```python
from build123d import *

# Parameters (mm, degrees)
SKETCH1_R           = 2.992461664
BOSS_EXTRUDE1_DEPTH = 8
CHAMFER2_SIZE       = 0.3


with BuildPart() as part:
    # Sketch1 → Boss-Extrude1 (new body)
    with BuildSketch(Plane(origin=(0, 0, 0), x_dir=(1, 0, 0), z_dir=(0, 1, 0))):
        Circle(SKETCH1_R)
        with BuildLine():
            Line((-1.125, 1.307669683), (-1.125, -1.307669683))
            ThreePointArc((-1.125, -1.307669683), (1.725, 0), (-1.125, 1.307669683))
        make_face(mode=Mode.SUBTRACT)
    extrude(amount=BOSS_EXTRUDE1_DEPTH)

    # Chamfer2
    chamfer2_edges = [part.edges().sort_by_distance(p)[0] for p in [
        (1.725, 8, 0),
        (-1.125, 8, 0),
    ]]
    chamfer(chamfer2_edges, length=CHAMFER2_SIZE)


solid = part.part
```
The model under review builds one solid part; all positions refer to its coordinate system, in mm. Coordinates: 2 decimals unless noted, no trailing zeros. Write each loop counter-clockwise with the first axis right and the second up, starting at its lowest first coordinate (ties: lowest second). Pieces come first, ordered by that corner, then holes.
1) We need section B-B on x = 0. State the section outline as (y, z) points (3 decimals).
2) We need section A-A on z = 0. State the section outline as (x, y) points (3 decimals).
3) We need section C-C on y = 3. State the section outline as (x, z) points (3 decimals), then the cut area to 3 significant figures.
4) To check wall thickness, follow probe 1 along Z at (x, y) = (0, 4.75) (3 decimals); probe 2 along X at (y, z) = (5.25, 0) (3 decimals); probe 3 along X at (y, z) = (7.5, -1.4). State the ranges of each line that lie inside material, in increasing order.
5) The part is to be moulded in two halves that separate along X. For faces 1 (the face through (2, 8, 1)), 2 (the face through (-1.125, 4, 0)), 3 (the face through (2.854, 3.944, -0.899)), say which applies: pulls with the +X half, pulls with the -X half, needs draft (parallel to the pull), parting line crosses it, or undercut.
6) Clearance check with a flat-ended pin moving along its axis: pin 1 Ø1 at (y, z) = (6, 2) entering from +X. State where the tip first meets the part, or that it passes through.
7) We need section D-D on z = 2.65. State the section outline as (x, y) points, then the cut area to 3 significant figures.
Answer list:
1. outline: (0, -2.992) - (8, -2.992) - (8, -2.025) - (7.7, -1.725) - (0, -1.725) - close; (0, 1.725) - (7.7, 1.725) - (8, 2.025) - (8, 2.992) - (0, 2.992) - close
2. outline: (-2.992, 0) - (-1.125, 0) - (-1.125, 7.7) - (-1.425, 8) - (-2.992, 8) - close; (1.725, 0) - (2.992, 0) - (2.992, 8) - (2.025, 8) - (1.725, 7.7) - close
3. outline: circle Ø5.985 at (0, 0); hole (-1.125, -1.308) arc R1.725 ccw (long way) to (-1.125, 1.308) - close
3. area: 19.9 mm2
4. probe 1: z = -2.992 to -1.725, 1.725 to 2.992
4. probe 2: x = -2.992 to -1.125, 1.725 to 2.992
4. probe 3: x = -2.64 to -1.01, 1.01 to 2.64
5. face 1: needs draft
5. face 2: undercut
5. face 3: parting line crosses it
6. pin 1: stops at x = 2.59
7. outline: (-1.39, 0) - (1.39, 0) - (1.39, 8) - (-1.39, 8) - close
7. area: 22.2 mm2
